Can you work these out from the model? Positions are in its coordinate system, mm. A direction names the side the tool comes from. Give positions to 0.01 mm unless a question says otherwise; leave off trailing zeros. Loops run counter-clockwise (first coordinate to the right, second up) from the corner with the lowest first, then second, coordinate; pieces in that order, holes last. Notation, with made-up numbers: M -37,86 L 18,86 A21 cw 18,94 Z; hole C -6.75,11 d2. An arc over 180 degrees is marked long. Use CSV: the item, a comma, the result in double quotes.
from build123d import *

# Parameters (mm, degrees)
F0_W          = 50.292
F0_H          = 82.042
F1_DEPTH      = 48.006
F2_W          = 39.4548750482
F2_H          = 39.4502789713
F3_DEPTH      = 101.6
F4_W          = 71.629058104
F4_H          = 39.4502789713
F5_DEPTH      = 101.6
F5_DEPTH_BACK = 25.4
F6_T1_DEPTH   = 5.7536101086
F6_T3_DEPTH   = 5.0835148431
F6_T8_DEPTH   = 58.0102084241
F6_T14_DEPTH  = 58.0102084241
F6_T20_DEPTH  = 58.0102084241
F6_T26_DEPTH  = 57.3401131586
F6_T32_DEPTH  = 57.3401131586
F6_T38_DEPTH  = 58.0102084241
F6_T44_DEPTH  = 57.3401131586
F6_T50_DEPTH  = 57.3401131586
F7_W          = 4.0118359902
F7_H          = 8.2200020552
F8_DEPTH      = 19.05
F9_DEPTH      = 12.7
F10_SIZE      = 19.04999
F11_DEPTH     = 5.08
F13_DEPTH     = 10.16
F14_W         = 18.1836719804
F14_H         = 16.51
F15_DEPTH     = 10.16
F16_R         = 5.08
F17_DEPTH     = 5.08
F18_W         = 38.7847797828
F18_H         = 3.7839086726
F19_DEPTH     = 40.64


# Not quite as in the source:
# - a fillet or chamfer that OpenCascade refuses, or shapes differently, is made with other operations: its cross-section is extruded or revolved along the edge and cut away or added
# - a fillet or chamfer is up to 0.001 mm smaller than in the source, because OpenCascade refuses the exact size


with BuildPart() as f1:
    # F0 (on Top) → F1 (new body)
    with BuildSketch(Plane.XY):
        with Locations((25.146, 41.021)):
            Rectangle(F0_W, F0_H)
    extrude(amount=F1_DEPTH)

    # F2 (on face) → F3 (cut)
    with BuildSketch(Plane.XZ):
        with Locations((24.8109523673, 23.683816893)):
            Rectangle(F2_W, F2_H)
    extrude(amount=-F3_DEPTH, mode=Mode.SUBTRACT)

    # F4 (on face) → F5 (cut, two sides)
    with BuildSketch(Plane.YZ.offset(5.0835148431)) as f5_sk:
        with Locations((41.033150861, 23.683816893)):
            Rectangle(F4_W, F4_H)
    extrude(amount=F5_DEPTH, mode=Mode.SUBTRACT)
    extrude(f5_sk.sketch, amount=-F5_DEPTH_BACK, mode=Mode.SUBTRACT)

    # F6: chamfer of 20.32 on 8 edges, made by hand

    # F6_s2 → F6_t1 (join)
    with BuildSketch(Plane.YZ.offset(44.5383898914)):
        Polygon((56.527679913, 3.9586774074), (76.847679913, 24.2786774074), (76.847679913, 3.9586774074), align=None)
        Polygon((25.538621809, 3.9586774074), (5.218621809, 24.2786774074), (5.218621809, 3.9586774074), align=None)
        Polygon((25.538621809, 43.4089563787), (5.218621809, 23.0889563787), (5.218621809, 43.4089563787), align=None)
        Polygon((56.527679913, 43.4089563787), (76.847679913, 23.0889563787), (76.847679913, 43.4089563787), align=None)
    extrude(amount=F6_T1_DEPTH)

    # F6_s4 → F6_t3 (join)
    with BuildSketch(Plane.YZ):
        Polygon((25.538621809, 43.4089563787), (5.218621809, 23.0889563787), (5.218621809, 43.4089563787), align=None)
        Polygon((25.538621809, 3.9586774074), (5.218621809, 24.2786774074), (5.218621809, 3.9586774074), align=None)
        Polygon((76.847679913, 23.0889563787), (56.527679913, 43.4089563787), (76.847679913, 43.4089563787), align=None)
        Polygon((56.527679913, 3.9586774074), (76.847679913, 24.2786774074), (76.847679913, 3.9586774074), align=None)
    extrude(amount=F6_T3_DEPTH)


with BuildPart() as f6_tool6:
    # F6_s7 → F6_t8 (new body)
    with BuildSketch(Plane.YZ.offset(-7.7182084241)):
        Polygon((56.527679913, 3.9586774074), (76.847679913, 24.2786774074), (76.847679913, 3.9586774074), align=None)
    extrude(amount=F6_T8_DEPTH)

    split(bisect_by=Plane.YZ, keep=Keep.TOP)

    split(bisect_by=Plane.YZ.offset(5.0835148431), keep=Keep.BOTTOM)


with BuildPart() as f1_1:
    add(f1.part)

    # F6_t5: union F6_tool6
    add(f6_tool6.part)


with BuildPart() as f6_tool12:
    # F6_s13 → F6_t14 (new body)
    with BuildSketch(Plane.YZ.offset(-7.7182084241)):
        Polygon((25.538621809, 3.9586774074), (5.218621809, 24.2786774074), (5.218621809, 3.9586774074), align=None)
    extrude(amount=F6_T14_DEPTH)

    split(bisect_by=Plane.YZ, keep=Keep.TOP)

    split(bisect_by=Plane.YZ.offset(5.0835148431), keep=Keep.BOTTOM)


with BuildPart() as f1_2:
    add(f1_1.part)

    # F6_t11: union F6_tool12
    add(f6_tool12.part)


with BuildPart() as f6_tool18:
    # F6_s19 → F6_t20 (new body)
    with BuildSketch(Plane.YZ.offset(50.292)):
        Polygon((25.538621809, 43.4089563787), (5.218621809, 23.0889563787), (5.218621809, 43.4089563787), align=None)
    extrude(amount=-F6_T20_DEPTH)

    split(bisect_by=Plane.YZ, keep=Keep.TOP)

    split(bisect_by=Plane.YZ.offset(5.0835148431), keep=Keep.BOTTOM)


with BuildPart() as f1_3:
    add(f1_2.part)

    # F6_t17: union F6_tool18
    add(f6_tool18.part)


with BuildPart() as f6_tool24:
    # F6_s25 → F6_t26 (new body)
    with BuildSketch(Plane.YZ.offset(57.3401131586)):
        Polygon((25.538621809, 43.4089563787), (5.218621809, 23.0889563787), (5.218621809, 43.4089563787), align=None)
    extrude(amount=-F6_T26_DEPTH)

    split(bisect_by=Plane.YZ.offset(50.292), keep=Keep.BOTTOM)

    split(bisect_by=Plane.YZ.offset(44.5383898914), keep=Keep.TOP)


with BuildPart() as f1_4:
    add(f1_3.part)

    # F6_t23: union F6_tool24
    add(f6_tool24.part)


with BuildPart() as f6_tool30:
    # F6_s31 → F6_t32 (new body)
    with BuildSketch(Plane.YZ):
        Polygon((25.538621809, 3.9586774074), (5.218621809, 24.2786774074), (5.218621809, 3.9586774074), align=None)
    extrude(amount=F6_T32_DEPTH)

    split(bisect_by=Plane.YZ.offset(50.292), keep=Keep.BOTTOM)

    split(bisect_by=Plane.YZ.offset(44.5383898914), keep=Keep.TOP)


with BuildPart() as f1_5:
    add(f1_4.part)

    # F6_t29: union F6_tool30
    add(f6_tool30.part)


with BuildPart() as f6_tool36:
    # F6_s37 → F6_t38 (new body)
    with BuildSketch(Plane.YZ.offset(50.292)):
        Polygon((56.527679913, 43.4089563787), (76.847679913, 23.0889563787), (76.847679913, 43.4089563787), align=None)
    extrude(amount=-F6_T38_DEPTH)

    split(bisect_by=Plane.YZ, keep=Keep.TOP)

    split(bisect_by=Plane.YZ.offset(5.0835148431), keep=Keep.BOTTOM)


with BuildPart() as f1_6:
    add(f1_5.part)

    # F6_t35: union F6_tool36
    add(f6_tool36.part)


with BuildPart() as f6_tool42:
    # F6_s43 → F6_t44 (new body)
    with BuildSketch(Plane.YZ.offset(57.3401131586)):
        Polygon((76.847679913, 23.0889563787), (56.527679913, 43.4089563787), (76.847679913, 43.4089563787), align=None)
    extrude(amount=-F6_T44_DEPTH)

    split(bisect_by=Plane.YZ.offset(50.292), keep=Keep.BOTTOM)

    split(bisect_by=Plane.YZ.offset(44.5383898914), keep=Keep.TOP)


with BuildPart() as f1_7:
    add(f1_6.part)

    # F6_t41: union F6_tool42
    add(f6_tool42.part)


with BuildPart() as f6_tool48:
    # F6_s49 → F6_t50 (new body)
    with BuildSketch(Plane.YZ):
        Polygon((56.527679913, 3.9586774074), (76.847679913, 24.2786774074), (76.847679913, 3.9586774074), align=None)
    extrude(amount=F6_T50_DEPTH)

    split(bisect_by=Plane.YZ.offset(50.292), keep=Keep.BOTTOM)

    split(bisect_by=Plane.YZ.offset(44.5383898914), keep=Keep.TOP)


with BuildPart() as f1_8:
    add(f1_7.part)

    # F6_t47: union F6_tool48
    add(f6_tool48.part)

    # F7 (on face) → F8 (join)
    with BuildSketch(Plane.XY.offset(48.006)):
        with Locations((27.1519179951, 36.1947827041)):
            Rectangle(F7_W, F7_H)
    extrude(amount=F8_DEPTH)

    # F9 (add): a face of the model
    f9_faces = [f1_8.faces().sort_by_distance(p)[0] for p in [
        (27.1519179951, 40.3047837317, 57.531),
    ]]
    extrude(f9_faces, amount=F9_DEPTH)

    # F10 (size 19.05 in the source; OpenCascade refuses exactly that, so slightly less here)
    f10_edges = [f1_8.edges().sort_by_distance(p)[0] for p in [
        (27.151918, 32.084782, 67.056),
    ]]
    chamfer(f10_edges, length=F10_SIZE)

    # F11 (add): a face of the model
    f11_faces = [f1_8.faces().sort_by_distance(p)[0] for p in [
        (29.1578359902, 45.9802990729, 54.8770427375),
    ]]
    extrude(f11_faces, amount=F11_DEPTH)

    # F12: F1 across face


with BuildPart() as f1_9:
    add(f1_8.part)
    add(f1_8.part.mirror(Plane(origin=(25.146, 45.9802990729, 54.8770427375), x_dir=(0, -1, 0), z_dir=(-1, 0, 0))))

    # F13 (add): a face of the model
    f13_faces = [f1_9.faces().sort_by_distance(p)[0] for p in [
        (25.146, 53.0047837317, 57.531),
    ]]
    extrude(f13_faces, amount=F13_DEPTH)

    # F14 (on face) → F15 (cut)
    with BuildSketch(Plane(origin=(0, 63.1647837317, 0), x_dir=(-1, 0, 0), z_dir=(0, 1, 0))):
        with Locations((-25.146, 56.261)):
            Rectangle(F14_W, F14_H)
    extrude(amount=-F15_DEPTH, mode=Mode.SUBTRACT)

    # F16
    f16_edges = [f1_9.edges().sort_by_distance(p)[0] for p in [
        (25.146, 53.004784, 64.516),
        (25.146, 53.004784, 48.006),
    ]]
    fillet(f16_edges, radius=F16_R)

    # F17 (add): a face of the model
    f17_faces = [f1_9.faces().sort_by_distance(p)[0] for p in [
        (25.146, 63.1647837317, 65.786),
    ]]
    extrude(f17_faces, amount=F17_DEPTH)

    # F18 (on face) → F19 (join)
    with BuildSketch(Plane.XY.offset(3.9586774074)):
        with Locations((25.146, 1.8919543363)):
            Rectangle(F18_W, F18_H)
    extrude(amount=F19_DEPTH)


solid = f1_9.part
Q1. For faces 1 (the flat face through (2.837, 66.528, 33.408)), 2 (the flat face through (25, 68.245, 66)), 3 (the cylindrical face through (25.019, 54.532, 63.067)), 4 (the flat face through (16.054, 46, 55)), which set-ups out of +Z, -Z, +X, -X, +Y, -Y let a thin tool reach every point of the face, with its end or its side?
Model answer:
face 1,"+X, -X"
face 2,"+Z, +X, -X, +Y"
face 3,"+X, -X, +Y"
face 4,"+Z, -X, +Y, -Y"
Q2. If we mould it in two halves opening along Z, with no side actions, what happens to faces 5 (the flat face through (25, 42, 0)), 6 (the flat face through (47.37, 15.81, 33.68)), 7 (the cylindrical face through (25.019, 54.532, 49.455)), 8 (the flat face through (25, 82.042, 45))? For each: released by +Z, released by -Z, zero draft, split by the parting line, or undercut.
Model answer:
face 5,"released by -Z"
face 6,"undercut"
face 7,"undercut"
face 8,"zero draft"
Q3. I'm going to push flat-ended pins straight in: P1, Ø15, axis at y = 43, z = 61, coming from the -X side; P2, Ø0.8, axis at x = 28, z = 66, coming from the +Y side; P3, Ø1.9, axis at x = 29, z = 57, coming from the +Y side. Where does each tip first touch, or does it pass through?
Model answer:
P1,"x = 16.05"
P2,"y = 68.24"
P3,"y = 53"
Q4. I want a section at B-B, the plane z = 19.5. Please give me the cut outline in (x, y).
Model answer:
outline,"M 0,0 L 50.29,0 L 50.29,10 L 44.54,10 L 44.54,3.78 L 5.75,3.78 L 5.75,10 L 0,10 Z; M 0,72.07 L 5.75,72.07 L 5.75,82.04 L 0,82.04 Z; M 44.54,72.07 L 50.29,72.07 L 50.29,82.04 L 44.54,82.04 Z"
Q5. I want a section at A-A, the plane y = 28. Please give me the cut outline in (x, z), then the cut area to 3 significant figures.
Model answer:
outline,"M 0,0 L 50.29,0 L 50.29,3.96 L 0,3.96 Z; M 0,43.41 L 50.29,43.41 L 50.29,48.01 L 0,48.01 Z"
area,"430 mm2"
Q6. Please list where these lines run through material, in increasing order: L1, parallel to Z at x = 18, y = 58; L2, parallel to X at y = 63.5, z = 4; L3, parallel to Z at x = 15, y = 30. Write a range as from..to.
Model answer:
L1,"0..3.96, 43.41..48.01, 64.52..67.06"
L2,"0..5.75, 44.54..50.29"
L3,"0..3.96, 43.41..48.01"
Q7. I want a section at C-C, the plane x = 28. Please give me the cut outline in (y, z), then the cut area to 3 significant figures.
Model answer:
outline,"M 0,0 L 82.04,0 L 82.04,3.96 L 3.78,3.96 L 3.78,43.41 L 82.04,43.41 L 82.04,48.01 L 58.08,48.01 A5.08 cw 53,53.09 L 53,59.44 A5.08 cw 58.08,64.52 L 68.24,64.52 L 68.24,67.06 L 51.13,67.06 L 32.08,48.01 L 0,48.01 Z"
area,"1,120 mm2"
Q8. I want a section at D-D, the plane y = 61. Please give me the cut outline in (x, z).
Model answer:
outline,"M 0,0 L 50.29,0 L 50.29,8.43 L 44.54,8.43 L 44.54,3.96 L 5.75,3.96 L 5.75,8.43 L 0,8.43 Z; M 0,38.94 L 5.75,38.94 L 5.75,43.41 L 44.54,43.41 L 44.54,38.94 L 50.29,38.94 L 50.29,48.01 L 0,48.01 Z; M 16.05,64.52 L 34.24,64.52 L 34.24,67.06 L 16.05,67.06 Z"
